from build123d import *

# Parameters (mm, degrees)
SKETCH1_R           = 25
BOSS_EXTRUDE1_DEPTH = 45
SKETCH2_R           = 20
CUT_EXTRUDE1_DEPTH  = 17
SKETCH3_R           = 12.7
CUT_EXTRUDE2_DEPTH  = 18
SKETCH4_R           = 2
CUT_EXTRUDE3_DEPTH  = 46.099889135
CIRPATTERN1_COUNT   = 10
CUT_EXTRUDE4_START  = -20
SKETCH5_R           = 20
CUT_EXTRUDE4_DEPTH  = 20
CUT_EXTRUDE5_DEPTH  = 58.227615711


with BuildPart() as part:
    # Sketch1 → Boss-Extrude1 (new body)
    with BuildSketch(Plane.XY):
        with Locations(Location((0, 0, 0), (0, 0, 180))):
            Circle(SKETCH1_R)
    extrude(amount=BOSS_EXTRUDE1_DEPTH)

    # Sketch2 → Cut-Extrude1 (cut)
    with BuildSketch(Plane.XY.offset(45)):
        Circle(SKETCH2_R)
    extrude(amount=-CUT_EXTRUDE1_DEPTH, mode=Mode.SUBTRACT)

    # Sketch3 → Cut-Extrude2 (cut)
    with BuildSketch(Plane.XY.offset(28)):
        Circle(SKETCH3_R)
    extrude(amount=-CUT_EXTRUDE2_DEPTH, mode=Mode.SUBTRACT)

    # Sketch4 → Cut-Extrude3 (cut, through all)
    with BuildSketch(Plane.XY.offset(28)):
        with Locations((-7.552723676, 14.669913602)):
            Circle(SKETCH4_R)
    cut_extrude3 = extrude(amount=-CUT_EXTRUDE3_DEPTH, mode=Mode.SUBTRACT)

    # CirPattern1: Cut-Extrude3 ×10 about axis
    cirpattern1_axis = Axis((0, 0, 0), (0, 0, 1))
    for i in range(1, CIRPATTERN1_COUNT):
        add(cut_extrude3.rotate(cirpattern1_axis, i * 360 / CIRPATTERN1_COUNT), mode=Mode.SUBTRACT)

    # Sketch5 → Cut-Extrude4 (cut)
    with BuildSketch(Plane(origin=(0, 0, 0), x_dir=(-1, 0, 0), z_dir=(0, 0, -1)).offset(CUT_EXTRUDE4_START)):
        with Locations(Location((0, 0, 0), (0, 0, 180))):
            Circle(SKETCH5_R)
    extrude(amount=CUT_EXTRUDE4_DEPTH, mode=Mode.SUBTRACT)

    # Sketch6 → Cut-Extrude5 (cut, through all)
    with BuildSketch(Plane(origin=(0, 0, 0), x_dir=(-1, 0, 0), z_dir=(0, 0, -1))):
        with BuildLine():
            Line((-8.8, 23.4), (8.8, 23.4))
            ThreePointArc((8.8, 23.4), (0, 25), (-8.8, 23.4))
        make_face()
        with BuildLine():
            Line((-8.8, -23.4), (8.8, -23.4))
            ThreePointArc((8.8, -23.4), (0, -25), (-8.8, -23.4))
        make_face()
    extrude(amount=-CUT_EXTRUDE5_DEPTH, mode=Mode.SUBTRACT)


solid = part.part
Here's how the part is built. I have some questions about the finished solid (model axes, mm). A direction names the side the tool comes from. Round coordinates to 2 decimals unless told otherwise and drop trailing zeros. Order: outer loops, then holes, each group sorted by start corner. A loop starts at its lowest first (then second) coordinate and runs counter-clockwise, first axis right, second up. Notation, with made-up numbers: M -21.75,-36.5 L -15.75,-36.5 A33 ccw -15.75,2.5 Z; hole C 31.25,10.25 d2. An arc over 180 degrees is marked long. Return JSON: item names as keys, results as strings. Group by question number.
1. I'm going to push flat-ended pins straight in: pin 1 Ø6 at (x, y) = (0.5, -10) entering from +Z; pin 2 Ø1.5 at (x, z) = (11.5, 39.5) entering from +Y; pin 3 Ø6.5 at (x, y) = (-16.29, -2.65) entering from -Z. Where does each tip first touch, or does it pass through?
2. On a 3-axis mill with a long thin cutter (end or side, diameter ignored), from which of +Z, -Z, +X, -X, +Y, -Y can I reach the whole of each face in a straight line? I mean faces 4 (the face through (-19.98, -0.88, 10.14)), 5 (the face through (13, 0, 28)), 6 (the face through (-12.78, -10.09, 24.06)). Say none if no direction works.
3. If we section it at D-D on y = -3.5: List the corners of the cut face in (x, z) for me.
4. If we section it at A-A on z = 12: List the corners of the cut face in (x, y) for me, then the cut area to 3 significant figures.
5. If we mould it in two halves opening along Y, with no side actions, what happens to faces 1 (the face through (-16.11, 8.88, 24.06)), 2 (the face through (-13, -16, 45)), 3 (the face through (0, 23.4, 22))? For each: pulls with the +Y half, pulls with the -Y half, needs draft (parallel to the pull), parting line crosses it, or undercut.
6. If we section it at B-B on y = 2.5: List the corners of the cut face in (x, z) for me, then the cut area to 3 significant figures.
7. If we section it at C-C on z = 24: State how many separate pieces and enclosed holes the cut face has, then the cut area to 3 significant figures.
8. Please list where these lines run through material, in increasing order: probe 1 along Y at (x, z) = (0, 6.25); probe 2 along X at (y, z) = (-4, 23); probe 3 along X at (y, z) = (1, 22.5).
Reply:
{
 "1": {"pin 1": "z = 28", "pin 2": "y = 22.57", "pin 3": "z = 20"},
 "2": {"face 4": "-Z", "face 5": "+Z", "face 6": "+Z, -Z"},
 "3": {"outline": "M -24.75,0 L -19.69,0 L -19.69,20 L -18.1,20 L -18.1,28 L -19.69,28 L -19.69,45 L -24.75,45 Z; M -14.48,20 L -12.21,20 L -12.21,28 L -14.48,28 Z; M 12.21,20 L 19.69,20 L 19.69,0 L 24.75,0 L 24.75,45 L 19.69,45 L 19.69,28 L 12.21,28 Z"},
 "4": {"outline": "M -8.8,-23.4 L 8.8,-23.4 A25 ccw 8.8,23.4 L -8.8,23.4 A25 ccw Z; hole C 0,0 d40", "area": "669 mm^2"},
 "5": {"face 1": "undercut", "face 2": "needs draft", "face 3": "pulls with the +Y half"},
 "6": {"outline": "M -24.87,0 L -19.84,0 L -19.84,20 L -12.45,20 L -12.45,28 L -19.84,28 L -19.84,45 L -24.87,45 Z; M 12.45,20 L 14.29,20 L 14.29,28 L 12.45,28 Z; M 18.28,20 L 19.84,20 L 19.84,0 L 24.87,0 L 24.87,45 L 19.84,45 L 19.84,28 L 18.28,28 Z", "area": "539 mm^2"},
 "7": {"separate pieces": "1", "enclosed holes": "11", "area": "1,290 mm^2"},
 "8": {"probe 1": "-23.4 to -20, 20 to 23.4", "probe 2": "-24.68 to -17.76, -14.81 to -12.05, 12.05 to 24.68", "probe 3": "-24.98 to -12.66, 12.66 to 15.16, 17.42 to 24.98"}
}
